Build history of the part. All positions in model axes, mm. A direction names the side the tool comes from. Coordinates: 2 decimals unless noted, no trailing zeros. Loops run counter-clockwise (first coordinate to the right, second up) from the corner with the lowest first, then second, coordinate; pieces in that order, holes last. Notation, with made-up numbers: (29.25, 23) -> (68.25, 23) arc R9 cw to (68.25, 32) -> close; hole circle Ø5 at (-37, -34). An arc over 180 degrees is marked (long way). One line per item, written item: value. Start each with the question number.
```python
from build123d import *

# Parameters (mm, degrees)
F1_DEPTH      = 52
F1_DEPTH_BACK = 52
F0_W          = 95
F0_H          = 460.873763546
F2_DEPTH      = 45
F2_DEPTH_BACK = 45
F3_R          = 30
F4_T1_DEPTH   = 104
F5_T1_DEPTH   = 104
F6_SIZE       = 10
F7_W          = 90
F7_H          = 95
F8_DEPTH      = 50
F9_W          = 90
F9_H          = 95
F10_DEPTH     = 60
F11_T4_DEPTH  = 65.575795383
F11_T10_DEPTH = 65.575795383
F11_T16_DEPTH = 65.575795383
F11_T22_DEPTH = 65.575795383
F11_T28_DEPTH = 65.575795383
F11_T34_DEPTH = 65.575795383
F11_T40_DEPTH = 65.575795383
F11_T46_DEPTH = 65.575795383
F12_T4_DEPTH  = 65.575795383
F12_T10_DEPTH = 65.575795383
F12_T16_DEPTH = 65.575795383
F12_T22_DEPTH = 65.575795383
F12_T28_DEPTH = 65.575795383
F12_T34_DEPTH = 65.575795383
F12_T40_DEPTH = 65.575795383
F12_T46_DEPTH = 65.575795383
F13_R         = 2


# Not quite as in the source:
# - a fillet or chamfer that OpenCascade refuses, or shapes differently, is made with other operations: its cross-section is extruded or revolved along the edge and cut away or added


with BuildPart() as f1:
    # F0 (on Right) → F1 (new body, two sides)
    with BuildSketch(Plane.YZ) as f1_sk:
        Polygon((-405, 55), (-405, 0), (405, 0), (405, 55), (200, 55), (200, 110), (195, 110), (100, 110), (0, 110), (-100, 110), (-195, 110), (-200, 110), (-200, 55), align=None)
    extrude(amount=F1_DEPTH)
    extrude(f1_sk.sketch, amount=-F1_DEPTH_BACK)

    # F0 (on Right) → F2 (join, two sides)
    with BuildSketch(Plane.YZ) as f2_sk:
        with Locations((-147.5, 340.436881773)):
            Rectangle(F0_W, F0_H)
        with Locations((147.5, 340.436881773)):
            Rectangle(F0_W, F0_H)
    extrude(amount=-F2_DEPTH)
    extrude(f2_sk.sketch, amount=F2_DEPTH_BACK)

    # F3
    f3_edges = [f1.edges().sort_by_distance(p)[0] for p in [
        (0, 405, 55),
        (0, -405, 55),
    ]]
    fillet(f3_edges, radius=F3_R)

    # F4: fillet of radius 80 on 1 edges, made by hand

    # F4_s2 → F4_t1 (join)
    with BuildSketch(Plane.YZ.offset(-52)):
        with BuildLine():
            ThreePointArc((275.9934207679, 55), (229.0892631696, 70.1925930159), (200, 110))
            Line((200, 110), (200, 55))
            Line((200, 55), (275.9934207679, 55))
        make_face()
    extrude(amount=F4_T1_DEPTH)

    # F5: fillet of radius 80 on 1 edges, made by hand

    # F5_s2 → F5_t1 (join)
    with BuildSketch(Plane.YZ.offset(-52)):
        with BuildLine():
            ThreePointArc((-275.9934207679, 55), (-229.0892631696, 70.1925930159), (-200, 110))
            Line((-200, 110), (-200, 55))
            Line((-200, 55), (-275.9934207679, 55))
        make_face()
    extrude(amount=F5_T1_DEPTH)

    # F6
    f6_edges = [f1.edges().sort_by_distance(p)[0] for p in [
        (45, -195, 340.436882),
        (45, -100, 340.436882),
        (45, 100, 340.436882),
        (-45, -195, 340.436882),
        (-45, -100, 340.436882),
        (-45, 100, 340.436882),
        (-45, 195, 340.436882),
        (45, 195, 340.436882),
    ]]
    chamfer(f6_edges, length=F6_SIZE)

    # F7 (on face) → F8 (join)
    with BuildSketch(Plane.XY.offset(110)):
        with Locations((0, -147.5)):
            Rectangle(F7_W, F7_H)
        with Locations((0, 147.5)):
            Rectangle(F7_W, F7_H)
    extrude(amount=F8_DEPTH)

    # F9 (on face) → F10 (join)
    with BuildSketch(Plane.XY.offset(570.873763546)):
        Polygon((45, -110), (45, -100), (35, -100), align=None)
        Polygon((-45, -110), (-35, -100), (-45, -100), align=None)
        Polygon((45, -195), (45, -185), (35, -195), align=None)
        Polygon((-35, -195), (-45, -185), (-45, -195), align=None)
        with Locations((0, 147.5)):
            Rectangle(F9_W, F9_H)
        Polygon((45, -110), (35, -100), (-35, -100), (-45, -110), (-45, -185), (-35, -195), (35, -195), (45, -185), align=None)
    extrude(amount=-F10_DEPTH)

    # F11: chamfer of 10 on 8 edges, made by hand


with BuildPart() as f11_tool2:
    # F11_s3 → F11_t4 (new body)
    with BuildSketch(Plane(origin=(-98.1845447985, -98.1845447985, 0), x_dir=(0, 0, 1), z_dir=(0.7071067812, 0.7071067812, 0))):
        Polygon((510.873763546, 172.6345596729), (500.873763546, 162.6345596729), (510.873763546, 162.6345596729), align=None)
    extrude(amount=F11_T4_DEPTH)

    split(bisect_by=Plane.YZ.offset(45), keep=Keep.BOTTOM)

    split(bisect_by=Plane.XZ.offset(195), keep=Keep.BOTTOM)


with BuildPart() as f1_1:
    add(f1.part)

    # F11_t1: union F11_tool2
    add(f11_tool2.part)


with BuildPart() as f11_tool8:
    # F11_s9 → F11_t10 (new body)
    with BuildSketch(Plane(origin=(49.3154552015, -49.3154552015, 0), x_dir=(0, 0, 1), z_dir=(0.7071067812, -0.7071067812, 0))):
        Polygon((500.873763546, 45.9619407771), (510.873763546, 35.9619407771), (510.873763546, 45.9619407771), align=None)
    extrude(amount=F11_T10_DEPTH)

    split(bisect_by=Plane.YZ.offset(45), keep=Keep.BOTTOM)

    split(bisect_by=Plane.XZ.offset(100), keep=Keep.TOP)


with BuildPart() as f1_2:
    add(f1_1.part)

    # F11_t7: union F11_tool8
    add(f11_tool8.part)


with BuildPart() as f11_tool14:
    # F11_s15 → F11_t16 (new body)
    with BuildSketch(Plane(origin=(-95.6845447985, -95.6845447985, 0), x_dir=(0, 0, 1), z_dir=(0.7071067812, 0.7071067812, 0))):
        Polygon((510.873763546, 35.9619407771), (500.873763546, 45.9619407771), (510.873763546, 45.9619407771), align=None)
    extrude(amount=F11_T16_DEPTH)

    split(bisect_by=Plane.YZ.offset(-45), keep=Keep.TOP)

    split(bisect_by=Plane.XZ.offset(100), keep=Keep.TOP)


with BuildPart() as f1_3:
    add(f1_2.part)

    # F11_t13: union F11_tool14
    add(f11_tool14.part)


with BuildPart() as f11_tool20:
    # F11_s21 → F11_t22 (new body)
    with BuildSketch(Plane(origin=(98.1845447985, -98.1845447985, 0), x_dir=(0, 0, 1), z_dir=(-0.7071067812, 0.7071067812, 0))):
        Polygon((510.873763546, -172.6345596729), (500.873763546, -162.6345596729), (510.873763546, -162.6345596729), align=None)
    extrude(amount=F11_T22_DEPTH)

    split(bisect_by=Plane.XZ.offset(195), keep=Keep.BOTTOM)

    split(bisect_by=Plane.YZ.offset(-45), keep=Keep.TOP)


with BuildPart() as f1_4:
    add(f1_3.part)

    # F11_t19: union F11_tool20
    add(f11_tool20.part)


with BuildPart() as f11_tool26:
    # F11_s27 → F11_t28 (new body)
    with BuildSketch(Plane(origin=(-98.1845447985, 98.1845447985, 0), x_dir=(0, 0, 1), z_dir=(0.7071067812, -0.7071067812, 0))):
        Polygon((500.873763546, -162.6345596729), (510.873763546, -172.6345596729), (510.873763546, -162.6345596729), align=None)
    extrude(amount=F11_T28_DEPTH)

    split(bisect_by=Plane.YZ.offset(45), keep=Keep.BOTTOM)

    split(bisect_by=Plane.XZ.offset(-195), keep=Keep.TOP)


with BuildPart() as f1_5:
    add(f1_4.part)

    # F11_t25: union F11_tool26
    add(f11_tool26.part)


with BuildPart() as f11_tool32:
    # F11_s33 → F11_t34 (new body)
    with BuildSketch(Plane(origin=(49.3154552015, 49.3154552015, 0), x_dir=(0, 0, 1), z_dir=(0.7071067812, 0.7071067812, 0))):
        Polygon((510.873763546, -35.9619407771), (500.873763546, -45.9619407771), (510.873763546, -45.9619407771), align=None)
    extrude(amount=F11_T34_DEPTH)

    split(bisect_by=Plane.YZ.offset(45), keep=Keep.BOTTOM)

    split(bisect_by=Plane.XZ.offset(-100), keep=Keep.BOTTOM)


with BuildPart() as f1_6:
    add(f1_5.part)

    # F11_t31: union F11_tool32
    add(f11_tool32.part)


with BuildPart() as f11_tool38:
    # F11_s39 → F11_t40 (new body)
    with BuildSketch(Plane(origin=(-49.3154552015, 49.3154552015, 0), x_dir=(0, 0, 1), z_dir=(-0.7071067812, 0.7071067812, 0))):
        Polygon((510.873763546, 35.9619407771), (500.873763546, 45.9619407771), (510.873763546, 45.9619407771), align=None)
    extrude(amount=F11_T40_DEPTH)

    split(bisect_by=Plane.XZ.offset(-100), keep=Keep.BOTTOM)

    split(bisect_by=Plane.YZ.offset(-45), keep=Keep.TOP)


with BuildPart() as f1_7:
    add(f1_6.part)

    # F11_t37: union F11_tool38
    add(f11_tool38.part)


with BuildPart() as f11_tool44:
    # F11_s45 → F11_t46 (new body)
    with BuildSketch(Plane(origin=(51.8154552015, 51.8154552015, 0), x_dir=(0, 0, 1), z_dir=(0.7071067812, 0.7071067812, 0))):
        Polygon((510.873763546, -172.6345596729), (500.873763546, -162.6345596729), (510.873763546, -162.6345596729), align=None)
    extrude(amount=F11_T46_DEPTH)

    split(bisect_by=Plane.YZ.offset(-45), keep=Keep.TOP)

    split(bisect_by=Plane.XZ.offset(-195), keep=Keep.TOP)


with BuildPart() as f1_8:
    add(f1_7.part)

    # F11_t43: union F11_tool44
    add(f11_tool44.part)

    # F12: chamfer of 10 on 8 edges, made by hand


with BuildPart() as f12_tool2:
    # F12_s3 → F12_t4 (new body)
    with BuildSketch(Plane(origin=(51.8154552015, 51.8154552015, 0), x_dir=(0, 0, 1), z_dir=(0.7071067812, 0.7071067812, 0))):
        Polygon((170, -162.6345596729), (160, -172.6345596729), (160, -162.6345596729), align=None)
    extrude(amount=F12_T4_DEPTH)

    split(bisect_by=Plane.YZ.offset(-45), keep=Keep.TOP)

    split(bisect_by=Plane.XZ.offset(-195), keep=Keep.TOP)


with BuildPart() as f1_9:
    add(f1_8.part)

    # F12_t1: union F12_tool2
    add(f12_tool2.part)


with BuildPart() as f12_tool8:
    # F12_s9 → F12_t10 (new body)
    with BuildSketch(Plane(origin=(-98.1845447985, 98.1845447985, 0), x_dir=(0, 0, 1), z_dir=(0.7071067812, -0.7071067812, 0))):
        Polygon((160, -172.6345596729), (170, -162.6345596729), (160, -162.6345596729), align=None)
    extrude(amount=F12_T10_DEPTH)

    split(bisect_by=Plane.YZ.offset(45), keep=Keep.BOTTOM)

    split(bisect_by=Plane.XZ.offset(-195), keep=Keep.TOP)


with BuildPart() as f1_10:
    add(f1_9.part)

    # F12_t7: union F12_tool8
    add(f12_tool8.part)


with BuildPart() as f12_tool14:
    # F12_s15 → F12_t16 (new body)
    with BuildSketch(Plane(origin=(49.3154552015, 49.3154552015, 0), x_dir=(0, 0, 1), z_dir=(0.7071067812, 0.7071067812, 0))):
        Polygon((170, -45.9619407771), (160, -35.9619407771), (160, -45.9619407771), align=None)
    extrude(amount=F12_T16_DEPTH)

    split(bisect_by=Plane.YZ.offset(45), keep=Keep.BOTTOM)

    split(bisect_by=Plane.XZ.offset(-100), keep=Keep.BOTTOM)


with BuildPart() as f1_11:
    add(f1_10.part)

    # F12_t13: union F12_tool14
    add(f12_tool14.part)


with BuildPart() as f12_tool20:
    # F12_s21 → F12_t22 (new body)
    with BuildSketch(Plane(origin=(-98.1845447985, -98.1845447985, 0), x_dir=(0, 0, 1), z_dir=(0.7071067812, 0.7071067812, 0))):
        Polygon((170, 162.6345596729), (160, 172.6345596729), (160, 162.6345596729), align=None)
    extrude(amount=F12_T22_DEPTH)

    split(bisect_by=Plane.YZ.offset(45), keep=Keep.BOTTOM)

    split(bisect_by=Plane.XZ.offset(195), keep=Keep.BOTTOM)


with BuildPart() as f1_12:
    add(f1_11.part)

    # F12_t19: union F12_tool20
    add(f12_tool20.part)


with BuildPart() as f12_tool26:
    # F12_s27 → F12_t28 (new body)
    with BuildSketch(Plane(origin=(49.3154552015, -49.3154552015, 0), x_dir=(0, 0, 1), z_dir=(0.7071067812, -0.7071067812, 0))):
        Polygon((160, 35.9619407771), (170, 45.9619407771), (160, 45.9619407771), align=None)
    extrude(amount=F12_T28_DEPTH)

    split(bisect_by=Plane.YZ.offset(45), keep=Keep.BOTTOM)

    split(bisect_by=Plane.XZ.offset(100), keep=Keep.TOP)


with BuildPart() as f1_13:
    add(f1_12.part)

    # F12_t25: union F12_tool26
    add(f12_tool26.part)


with BuildPart() as f12_tool32:
    # F12_s33 → F12_t34 (new body)
    with BuildSketch(Plane(origin=(-95.6845447985, -95.6845447985, 0), x_dir=(0, 0, 1), z_dir=(0.7071067812, 0.7071067812, 0))):
        Polygon((170, 45.9619407771), (160, 35.9619407771), (160, 45.9619407771), align=None)
    extrude(amount=F12_T34_DEPTH)

    split(bisect_by=Plane.YZ.offset(-45), keep=Keep.TOP)

    split(bisect_by=Plane.XZ.offset(100), keep=Keep.TOP)


with BuildPart() as f1_14:
    add(f1_13.part)

    # F12_t31: union F12_tool32
    add(f12_tool32.part)


with BuildPart() as f12_tool38:
    # F12_s39 → F12_t40 (new body)
    with BuildSketch(Plane(origin=(-49.3154552015, 49.3154552015, 0), x_dir=(0, 0, 1), z_dir=(-0.7071067812, 0.7071067812, 0))):
        Polygon((170, 45.9619407771), (160, 35.9619407771), (160, 45.9619407771), align=None)
    extrude(amount=F12_T40_DEPTH)

    split(bisect_by=Plane.XZ.offset(-100), keep=Keep.BOTTOM)

    split(bisect_by=Plane.YZ.offset(-45), keep=Keep.TOP)


with BuildPart() as f1_15:
    add(f1_14.part)

    # F12_t37: union F12_tool38
    add(f12_tool38.part)


with BuildPart() as f12_tool44:
    # F12_s45 → F12_t46 (new body)
    with BuildSketch(Plane(origin=(98.1845447985, -98.1845447985, 0), x_dir=(0, 0, 1), z_dir=(-0.7071067812, 0.7071067812, 0))):
        Polygon((170, -162.6345596729), (160, -172.6345596729), (160, -162.6345596729), align=None)
    extrude(amount=F12_T46_DEPTH)

    split(bisect_by=Plane.XZ.offset(195), keep=Keep.BOTTOM)

    split(bisect_by=Plane.YZ.offset(-45), keep=Keep.TOP)


with BuildPart() as f1_16:
    add(f1_15.part)

    # F12_t43: union F12_tool44
    add(f12_tool44.part)

    # F13
    f13_edges = [f1_16.edges().sort_by_distance(p)[0] for p in [
        (52, -405, 12.5),
        (52, 0, 0),
        (52, 405, 12.5),
        (52, 396.213203, 46.213203),
        (52, 325.49671, 55),
        (52, 229.089263, 70.192593),
        (52, 0, 110),
        (52, -229.089263, 70.192593),
        (52, -325.49671, 55),
        (52, -396.213203, 46.213203),
        (-52, -405, 12.5),
        (-52, 0, 0),
        (-52, 405, 12.5),
        (-52, 396.213203, 46.213203),
        (-52, 325.49671, 55),
        (-52, 229.089263, 70.192593),
        (-52, 0, 110),
        (-52, -229.089263, 70.192593),
        (-52, -325.49671, 55),
        (-52, -396.213203, 46.213203),
    ]]
    fillet(f13_edges, radius=F13_R)


solid = f1_16.part
```
Item 1: Band-saw the part on B-B, the plane x = 16. List the corners of the cut face in (y, z).
Item 2: Probe probe 1 along Y at (x, z) = (-9, 438); probe 2 along X at (y, z) = (123, 407); probe 3 along Y at (x, z) = (-37, 405). List the from-to ranges inside material, lowest first.
Item 3: Drop flat-ended pins along their axis: pin 1 Ø2 at (x, y) = (26.5, -31) entering from +Z; pin 2 Ø1 at (x, y) = (35.5, -281) entering from +Z; pin 3 Ø10 at (x, z) = (39, 272.5) entering from -Y. Give the stop position or say it passes through.
Item 4: Two-plate mould, pull along Y, no slides. Class faces 1 (the face through (-0.7, -395.979, 46.445)), 2 (the face through (1, 3, 110)), 3 (the face through (45, -148, 344)), 4 (the face through (0.7, 395.979, 46.445)): +Y half, -Y half, draft (parallel to the pull), parting line (faces both ways), or undercut.
Item 5: Band-saw the part on C-C, the plane y = 139. List the corners of the cut face in (x, z), and give its area (3 significant figures).
Item 6: Tool access for faces 5 (the face through (45, 147, 344)), 6 (the face through (-1, 100, 344)), 7 (the face through (-45, -148, 344)), 8 (the face through (-1, -195, 344)): list every direction of +Z, -Z, +X, -X, +Y, -Y with a clear straight run to the whole face (end or side of a thin tool).
Item 7: Band-saw the part on D-D, the plane z = 135.5. List the corners of the cut face in (x, y), and give its area (3 significant figures).
Item 8: Band-saw the part on A-A, the plane z = 254.5. List the corners of the cut face in (x, y).
Worked out:
1. outline: (-405, 0) -> (405, 0) -> (405, 25) arc R30 ccw to (375, 55) -> (275.99, 55) arc R80 cw to (200, 110) -> (195, 110) -> (195, 570.87) -> (100, 570.87) -> (100, 110) -> (-100, 110) -> (-100, 570.87) -> (-195, 570.87) -> (-195, 110) -> (-200, 110) arc R80 cw to (-275.99, 55) -> (-375, 55) arc R30 ccw to (-405, 25) -> close
2. probe 1: y = -195 to -100, 100 to 195
2. probe 2: x = -45 to 45
2. probe 3: y = -193 to -102, 102 to 193
3. pin 1: stops at z = 110
3. pin 2: stops at z = 55
3. pin 3: stops at y = -195
4. face 1: -Y half
4. face 2: undercut
4. face 3: draft
4. face 4: +Y half
5. outline: (-52, 2) arc R2 ccw to (-50, 0) -> (50, 0) arc R2 ccw to (52, 2) -> (52, 108) arc R2 ccw to (50, 110) -> (45, 110) -> (45, 570.87) -> (-45, 570.87) -> (-45, 110) -> (-50, 110) arc R2 ccw to (-52, 108) -> close
5. area: 52,900 mm²
6. face 5: +Z, +X, +Y, -Y
6. face 6: +Z, +X, -X
6. face 7: +Z, -X, +Y, -Y
6. face 8: +Z, +X, -X, -Y
7. outline: (-45, -195) -> (45, -195) -> (45, -100) -> (-45, -100) -> close; (-45, 100) -> (45, 100) -> (45, 195) -> (-45, 195) -> close
7. area: 17,100 mm²
8. outline: (-45, -185) -> (-35, -195) -> (35, -195) -> (45, -185) -> (45, -110) -> (35, -100) -> (-35, -100) -> (-45, -110) -> close; (-45, 110) -> (-35, 100) -> (35, 100) -> (45, 110) -> (45, 185) -> (35, 195) -> (-35, 195) -> (-45, 185) -> close
